Part model, mm, in its own coordinate system. Face numbers are marked on the shaded views. A direction names the side the tool comes from. Coordinates: 2 decimals unless noted, no trailing zeros. Loops run counter-clockwise (first coordinate to the right, second up) from the corner with the lowest first, then second, coordinate; pieces in that order, holes last. Notation, with made-up numbers: (-10, 66.25) -> (28, 66.25) arc R14 ccw to (28, 76.25) -> close; hole circle Ø3 at (82, 26.25). An arc over 180 degrees is marked (long way). One line per question, with ' | ' between items. Start each with the question number.
1) Drop flat-ended pins along their axis: pin 1 (1 mm diameter, centred on x = -8.5, z = 0, fed in from -Y); pin 2 (1 mm diameter, centred on x = -9.5, z = -0.5, fed in from +Y); pin 3 (2 mm diameter, centred on y = -2, z = -3.5, fed in from -X). Give the stop position or say it passes through.
2) Cut at C-C (x = 7). List the corners of the cut face in (y, z), plus the area to 3 significant figures.
3) Two-plate mould, pull along X, no slides. Class the marked faces 3, 4 and 5: released by +X, released by -X, zero draft, split by the parting line, or undercut.
4) Cut at A-A (y = 0). Count the separate pieces of the cut face and the enclosed holes in it, plus the area to 3 significant figures.
5) 3-axis set-ups, long thin cutter, end or side, ignore diameter. For the marked faces 1 and 2: which of +Z, -Z, +X, -X, +Y, -Y reach the whole face in a straight line?
6) Cut at B-B (z = 0.5). List the corners of the cut face in (x, y).
7) Probe L1, parallel to X at y = -9.5, z = -0.75; L2, parallel to X at y = 5, z = -0.5; L3, parallel to X at y = 6, z = 4.5. List the from-to ranges inside material, lowest first. Write a range as from..to.
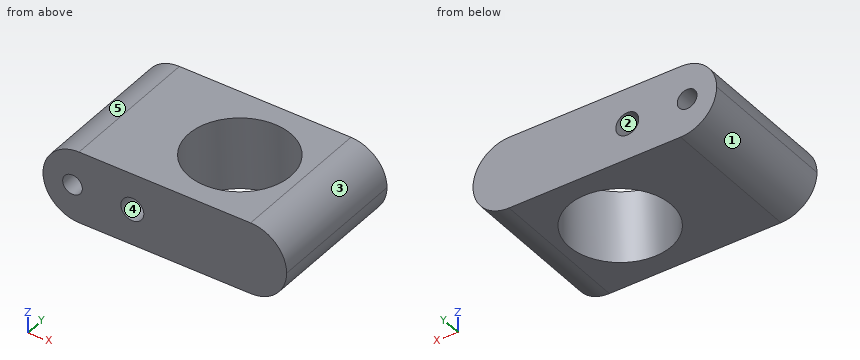
Autodesk Inventor part; units mm, degrees
ref_plane "YZ Plane" through (0, 0, 0) normal (1, 0, 0) x (0, 1, 0)
ref_plane "XZ Plane" through (0, 0, 0) normal (0, 1, 0) x (-1, 0, 0)
ref_plane "XY Plane" through (0, 0, 0) normal (0, 0, 1) x (1, 0, 0)
sketch "Sketch1" plane through (0, 0, 0) normal (0, 0, 1) x (1, 0, 0)
  circle A0 centre (0, 0) radius 7.8
  line L0 (0, 0) -> (-8.735, 0) construction
  line L1 (0, 0) -> (-17.865, 0) construction
  line L2 (-8.735, 0) -> (-8.735, 11) construction
  line L3 (-8.735, 0) -> (-8.735, -11) construction
  line L4 (-17.865, 0) -> (-17.865, -11) construction
  line L5 (-17.865, 0) -> (-17.865, 11) construction
  line L6 (7.8, 0) -> (14.8, 0) construction
  line L7 (-17.865, 0) -> (-22.365, 0) construction
  line L8 (-22.365, -11) -> (14.8, -11)
  line L9 (14.8, -11) -> (14.8, 11)
  line L10 (14.8, 11) -> (-22.365, 11)
  line L11 (-22.365, 11) -> (-22.365, -11)
  dimension "d0" = 15.6
  dimension "d1" = 8.735
  dimension "d2" = 17.865
  dimension "d3" = 11
  dimension "d4" = 11
  dimension "d5" = 11
  dimension "d6" = 11
  dimension "d7" = 7
  dimension "d8" = 4.5
  dimension "d23" = 37.165
extrude "Extrusion1" add sketch "Sketch1" along normal mid plane 11
sketch "Sketch2" plane through (-22.365, 11, 5.5) normal (0, 1, 0) x (1, 0, 0)
  line L0 (0, 11) -> (0, 0)
  line L1 (0, 5.5) -> (4.5, 5.5)
  line L2 (4.5, 5.5) -> (13.63, 5.5)
  circle A0 centre (4.5, 5.5) radius 1.5
  circle A1 centre (13.63, 5.5) radius 1.75
  point P0 (22.365, 5.5)
  dimension "d11" = 4.5
  dimension "d13" = 9.13
  dimension "d14" = 3
  dimension "d15" = 3.5
extrude "Extrusion2" cut sketch "Sketch2" against normal up to next contours A0 L2 L1 | L1 L2 A0
extrude "Extrusion3" cut sketch "Sketch2" against normal blind 4 contours A1
sketch "Sketch3" plane through (-22.365, -11, 5.5) normal (0, -1, 0) x (1, 0, 0)
  circle A0 centre (13.63, -5.5) radius 1.75
  circle A1 centre (13.63, -5.5) radius 1.75
  point P0 (22.365, -5.5)
extrude "Extrusion4" cut sketch "Sketch3" against normal blind 4
fillet "Fillet1" radius 5.5 4 edges at (-22.365, 0, 5.5) (14.8, 0, 5.5) (14.8, 0, -5.5) (-22.365, 0, -5.5)
equation "\"d23\" = d2 + d7 + 0.5 * d0 + d8"
properties part number "Reworked - PlateArmClip22mm"
Reported:
1) pin 1: stops at y = -7 | pin 2: stops at y = 7 | pin 3: stops at x = -21.76
2) outline: (-11, -5.5) -> (-3.44, -5.5) -> (-3.44, 5.5) -> (-11, 5.5) -> close; (3.44, -5.5) -> (11, -5.5) -> (11, 5.5) -> (3.44, 5.5) -> close | area: 166 mm²
3) face 3: released by +X | face 4: undercut | face 5: released by -X
4) separate pieces: 2 | enclosed holes: 1 | area: 204 mm²
5) face 1: -Z, -X, +Y, -Y | face 2: +Y
6) outline: (-22.34, -11) -> (-19.28, -11) -> (-19.28, 11) -> (-22.34, 11) -> close; (-16.45, -11) -> (-10.41, -11) -> (-10.41, -7) -> (-7.06, -7) -> (-7.06, -11) -> (14.78, -11) -> (14.78, 11) -> (-7.06, 11) -> (-7.06, 7) -> (-10.41, 7) -> (-10.41, 11) -> (-16.45, 11) -> close; hole circle Ø15.6 at (0, 0)
7) L1: x = -22.31..-19.16, -16.57..-10.32, -7.15..14.75 | L2: x = -22.34..-19.28, -16.45..-5.99, 5.99..14.78 | L3: x = -20.03..-4.98, 4.98..12.46
